Autodesk Inventor part; units mm, degrees
ref_plane "YZ Plane" through (0, 0, 0) normal (1, 0, 0) x (0, 1, 0)
ref_plane "XZ Plane" through (0, 0, 0) normal (0, 1, 0) x (-1, 0, 0)
ref_plane "XY Plane" through (0, 0, 0) normal (0, 0, 1) x (1, 0, 0)
sketch "Boceto1" plane through (0, 0, 0) normal (0, 0, 1) x (1, 0, 0)
  line L0 (5, 0) -> (30, 0)
  line L1 (35, 5) -> (35, 165)
  line L2 (30, 170) -> (5, 170)
  line L3 (0, 165) -> (0, 5)
  arc A0 (35, 165) -> (30, 170) centre (30, 165) ccw
  arc A1 (5, 170) -> (0, 165) centre (5, 165) ccw
  arc A2 (30, 0) -> (35, 5) centre (30, 5) ccw
  arc A3 (0, 5) -> (5, 0) centre (5, 5) ccw
extrude "Extrusión1" add sketch "Boceto1" against normal blind 3
sketch "Boceto2" plane through (0, 0, 0) normal (0, 0, 1) x (1, 0, 0)
  circle A0 centre (17.5, 140) radius 4.5
  circle A1 centre (29, 146.5) radius 1.25
  circle A2 centre (6, 146.5) radius 1.25
  circle A3 centre (6, 133) radius 1.25
  circle A4 centre (29, 133) radius 1.25
  circle A5 centre (17.5, 120) radius 2.5
  circle A6 centre (17.5, 100) radius 2.5
  circle A7 centre (17.5, 80) radius 2.5
  circle A8 centre (17.5, 20) radius 6.5
  circle A9 centre (12.5, 6) radius 2.5
  circle A10 centre (22.5, 6) radius 2.5
  circle A11 centre (12.5, 54.5) radius 2.5
  circle A12 centre (22.5, 54.5) radius 2.5
  point P0 (0, 0)
hole "Agujero1" at (17.5, 140, 0) direction (0, 0, -1) diameter 9 end through all
hole "Agujero2" at (29, 133, 0) at (29, 146.5, 0) at (6, 133, 0) at (6, 146.5, 0) direction (0, 0, -1) diameter 2.5 end through all
hole "Agujero3" at (17.5, 120, 0) at (17.5, 100, 0) at (17.5, 80, 0) at (22.5, 54.5, 0) at (12.5, 54.5, 0) at (22.5, 6, 0) at (12.5, 6, 0) direction (0, 0, -1) diameter 5 end through all
hole "Agujero4" at (17.5, 20, 0) direction (0, 0, -1) diameter 13 end through all
sketch "Boceto3" plane through (0, 0, -3) normal (0, 0, -1) x (-1, 0, 0)
  circle A0 centre (-17.5, 20) radius 6.5
  arc A1 (-27, 23.1225) -> (-8, 23.1225) centre (-17.5, 20) ccw
  line L0 (-17.5, 47) -> (-27, 47)
  line L1 (-17.5, 47) -> (-8, 47)
  line L2 (-8, 47) -> (-8, 23.1225)
  line L3 (-27, 47) -> (-27, 23.1225)
  point P0 (0, 0)
extrude "Extrusión2" cut sketch "Boceto3" against normal blind 10 contours A0 | L3 L0 L1 L2 A1
properties part number "1"
Read the model definition and answer for the solid it produces. Units are mm, in the model's axes. A direction names the side the tool comes from. Give positions to 0.01 mm unless a question says otherwise; leave off trailing zeros. Write each loop counter-clockwise with the first axis right and the second up, starting at its lowest first coordinate (ties: lowest second). Pieces come first, ordered by that corner, then holes. Notation, with made-up numbers: M 70.5,-37.5 L 117.5,-37.5 A20 ccw 117.5,-20.5 Z; hole C 58.25,-0.75 d8. An arc over 180 degrees is marked long. One line per item, written item: value. Start each with the question number.
(1) Find the intervals of material crossed by line 1 (X direction, y = 54.5, z = -0.9); line 2 (Y direction, x = 17.5, z = -2.2); line 3 (Y direction, x = 29, z = -0.85), in increasing order.
(2) Find section C-C (y = 20). Determine the outline of the cut face in (x, z), plus the area to 3 significant figures.
(3) Find section B-B (z = -1.9). Give the number of separate pieces and of enclosed holes in the cut face, plus the area to 3 significant figures.
(4) Determine the mould class of faces 1 (the flat face through (35, 84, -1)), 2 (the flat face through (17, 86, 0)), 3 (the flat face through (0, 86, -1)), 4 (the cylindrical face through (21.749, 52.115, -1.521)) for opening direction X: pulls with the +X half, pulls with the -X half, needs draft (parallel to the pull), parting line crosses it, or undercut.
(5) Find section D-D (y = 120). Determine the outline of the cut face in (x, z), plus the area to 3 significant figures.
(6) A tool of negligible diameter and unlimited length cuts with its end or side. For faces 5 (the cylindrical face through (34, 168, -1)), 6 (the flat face through (17, 47, -2)), from which of +Z, -Z, +X, -X, +Y, -Y can it reach the whole face along a straight path? Write none if from no direction.
(7) Find section A-A (y = 54.5). Determine the outline of the cut face in (x, z).
Results below:
1. line 1: x = 0 to 10, 15 to 20, 25 to 35
1. line 2: y = 0 to 10, 47 to 77.5, 82.5 to 97.5, 102.5 to 117.5, 122.5 to 135.5, 144.5 to 170
1. line 3: y = 0 to 131.75, 134.25 to 145.25, 147.75 to 170
2. outline: M 0,-3 L 7.5,-3 L 7.5,0 L 0,0 Z; M 27.5,-3 L 35,-3 L 35,0 L 27.5,0 Z
2. area: 45.0 mm^2
3. separate pieces: 1
3. enclosed holes: 13
3. area: 5,040 mm^2
4. face 1: pulls with the +X half
4. face 2: needs draft
4. face 3: pulls with the -X half
4. face 4: undercut
5. outline: M 0,-3 L 15,-3 L 15,0 L 0,0 Z; M 20,-3 L 35,-3 L 35,0 L 20,0 Z
5. area: 90.0 mm^2
6. face 5: +Z, -Z, +X, +Y
6. face 6: +Z, -Z
7. outline: M 0,-3 L 10,-3 L 10,0 L 0,0 Z; M 15,-3 L 20,-3 L 20,0 L 15,0 Z; M 25,-3 L 35,-3 L 35,0 L 25,0 Z
